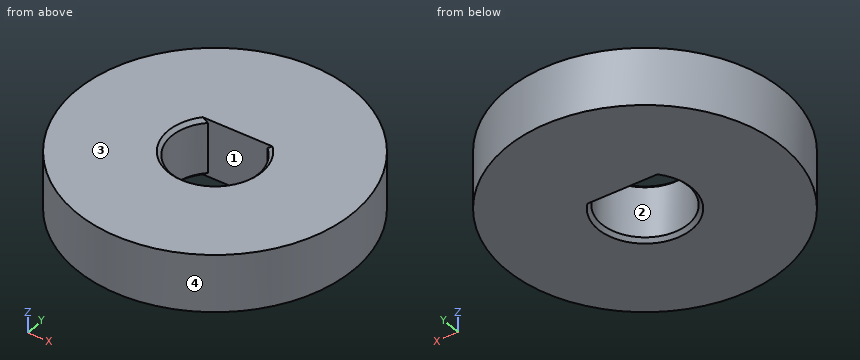
```python
from build123d import *

# Parameters (mm, degrees)
SKETCH1_R           = 30.48
SKETCH1_R_2         = 9.525
EXTRUDE1_DEPTH      = 6.35
CHAMFER1_SIZE       = 0.79375
BOSS_EXTRUDE1_DEPTH = 12.7


with BuildPart() as part:
    # Sketch1 → Extrude1 (new, symmetric)
    with BuildSketch(Plane.XY):
        Circle(SKETCH1_R)
        Circle(SKETCH1_R_2, mode=Mode.SUBTRACT)
    extrude(amount=EXTRUDE1_DEPTH, both=True)

    # Chamfer1
    chamfer1_edges = [part.edges().sort_by_distance(p)[0] for p in [
        (-9.525, 0, -6.35),
        (-9.525, 0, 6.35),
    ]]
    chamfer(chamfer1_edges, length=CHAMFER1_SIZE)

    # Sketch3 → Boss-Extrude1 (add, through all)
    with BuildSketch(Plane(origin=(0, 0, -6.35), x_dir=(-1, 0, 0), z_dir=(0, 0, -1))):
        with BuildLine():
            ThreePointArc((7.558172832, 7.025), (0, 10.31875), (-7.558172832, 7.025))
            Line((-7.558172832, 7.025), (7.558172832, 7.025))
        make_face()
    extrude(amount=-BOSS_EXTRUDE1_DEPTH)


solid = part.part
```
For this review, take the finished solid that the model builds, in its own axes (mm). Face numbers are marked on the shaded views. Round coordinates to 2 decimals unless told otherwise and drop trailing zeros. Write each loop counter-clockwise with the first axis right and the second up, starting at its lowest first coordinate (ties: lowest second). Pieces come first, ordered by that corner, then holes. Notation, with made-up numbers: (64.5, -27.5) - (85.5, -27.5) arc R23 cw to (85.5, -1.5) - close; hole circle Ø11 at (-38.5, 42). An arc over 180 degrees is marked (long way). Answer as CSV lines item,"result". Start each with the question number.
(1) Add section A-A, the plane x = 0. State the section outline as (y, z) points (3 decimals).
(2) Add section C-C, the plane z = -4.5. State the section outline as (x, y) points (3 decimals), plus the area to 3 significant figures.
(3) Add section B-B, the plane y = 0. State the section outline as (x, z) points (3 decimals), plus the area to 3 significant figures.
(4) Mouldability with a two-part tool opening along X and no side actions: class the marked faces 1, 2, 3 and 4 as +X half, -X half, draft (parallel to the pull), parting line (faces both ways), or undercut.
(5) Add section D-D, the plane y = 11. State the section outline as (x, z) points.
(6) For pin 1 (1.5 mm diameter, centred on y = 13, z = -3.5, fed in from +X); pin 2 (5 mm diameter, centred on y = -17.5, z = -1, fed in from +X), all flat-tipped, find the tip position at first contact; note any pin that passes through.
(7) For line 1 (Y direction, x = 0, z = 0) (3 decimals); line 2 (Y direction, x = 3, z = -0.75) (3 decimals); line 3 (X direction, y = 4.5, z = -0.75), list the stretches that pass through material, from the lowest coordinate up.
From the geometry:
1,outline,"(-30.48, -6.35) - (-10.319, -6.35) - (-9.525, -5.556) - (-9.525, 5.556) - (-10.319, 6.35) - (-30.48, 6.35) - close; (7.025, -6.35) - (30.48, -6.35) - (30.48, 6.35) - (7.025, 6.35) - close"
2,outline,"circle Ø60.96 at (0, 0); hole (-6.432, 7.025) arc R9.525 ccw (long way) to (6.432, 7.025) - close"
2,area,"2,660 mm²"
3,outline,"(-30.48, -6.35) - (-10.319, -6.35) - (-9.525, -5.556) - (-9.525, 5.556) - (-10.319, 6.35) - (-30.48, 6.35) - close; (9.525, -5.556) - (10.319, -6.35) - (30.48, -6.35) - (30.48, 6.35) - (10.319, 6.35) - (9.525, 5.556) - close"
3,area,"531 mm²"
4,face 1,"undercut"
4,face 2,"undercut"
4,face 3,"draft"
4,face 4,"parting line"
5,outline,"(-28.43, -6.35) - (28.43, -6.35) - (28.43, 6.35) - (-28.43, 6.35) - close"
6,pin 1,"stops at x = 27.91"
6,pin 2,"stops at x = 26.53"
7,line 1,"y = -30.48 to -9.525, 7.025 to 30.48"
7,line 2,"y = -30.332 to -9.04, 7.025 to 30.332"
7,line 3,"x = -30.15 to -8.39, 8.39 to 30.15"
